```python
from build123d import *

# Parameters (mm, degrees)
CYLINDER016_R     = 1.75
CYLINDER016_DEPTH = 22
CYLINDER017_R     = 3
CYLINDER017_DEPTH = 22
CYLINDER015_R     = 1.75
CYLINDER015_DEPTH = 22
CYLINDER014_R     = 3
CYLINDER014_DEPTH = 22
CYLINDER013_R     = 1.75
CYLINDER013_DEPTH = 22
CYLINDER012_R     = 3
CYLINDER012_DEPTH = 22
CYLINDER011_R     = 1.75
CYLINDER011_DEPTH = 22
CYLINDER010_R     = 3
CYLINDER010_DEPTH = 22
CYLINDER009_R     = 0.5
CYLINDER009_DEPTH = 2
CYLINDER008_R     = 0.5
CYLINDER008_DEPTH = 2
BOX002_W          = 17.5
BOX002_H          = 10
BOX002_DEPTH      = 5
CYLINDER006_R     = 0.93
CYLINDER006_DEPTH = 10
CYLINDER007_R     = 2
CYLINDER007_DEPTH = 10
CYLINDER005_R     = 0.93
CYLINDER005_DEPTH = 10
CYLINDER004_R     = 2
CYLINDER004_DEPTH = 10
CYLINDER003_R     = 0.93
CYLINDER003_DEPTH = 10
CYLINDER002_R     = 2
CYLINDER002_DEPTH = 10
CYLINDER001_R     = 0.93
CYLINDER001_DEPTH = 10
CYLINDER_R        = 2
CYLINDER_DEPTH    = 10
BOX001_W          = 46
BOX001_H          = 46
BOX001_DEPTH      = 25
BOX_W             = 50
BOX_H             = 50
BOX_DEPTH         = 25
FILLET_R          = 1.5
FILLET001_R       = 1
FILLET002_R       = 0.5


with BuildPart() as cylinder008:
    # Cylinder016 → Cylinder016 (new body)
    with BuildSketch(Plane.XY):
        Circle(CYLINDER016_R)
    extrude(amount=CYLINDER016_DEPTH)


with BuildPart() as cut008:
    # Cylinder017 → Cylinder017 (new body)
    with BuildSketch(Plane.XY):
        Circle(CYLINDER017_R)
    extrude(amount=CYLINDER017_DEPTH)

    # Cut008: cut Cylinder008
    add(cylinder008.part, mode=Mode.SUBTRACT)


with BuildPart() as cut008_1:
    # Cut008 placement: moved
    add(cut008.part.moved(Location((41, 35, 0))))


with BuildPart() as cylinder007:
    # Cylinder015 → Cylinder015 (new body)
    with BuildSketch(Plane.XY):
        Circle(CYLINDER015_R)
    extrude(amount=CYLINDER015_DEPTH)


with BuildPart() as fusion007:
    # Cylinder014 → Cylinder014 (new body)
    with BuildSketch(Plane.XY):
        Circle(CYLINDER014_R)
    extrude(amount=CYLINDER014_DEPTH)

    # Cut009: cut Cylinder007
    add(cylinder007.part, mode=Mode.SUBTRACT)


with BuildPart() as fusion007_1:
    # Cut009 placement: moved
    add(fusion007.part.moved(Location((6, 35, 0))))

    # Fusion007: union Cut008
    add(cut008_1.part)


with BuildPart() as fusion007_2:
    # Fusion007 placement: moved
    add(fusion007_1.part.moved(Location((0, -35, 0))))


with BuildPart() as cylinder005:
    # Cylinder013 → Cylinder013 (new body)
    with BuildSketch(Plane.XY):
        Circle(CYLINDER013_R)
    extrude(amount=CYLINDER013_DEPTH)


with BuildPart() as cut007:
    # Cylinder012 → Cylinder012 (new body)
    with BuildSketch(Plane.XY):
        Circle(CYLINDER012_R)
    extrude(amount=CYLINDER012_DEPTH)

    # Cut007: cut Cylinder005
    add(cylinder005.part, mode=Mode.SUBTRACT)


with BuildPart() as cut007_1:
    # Cut007 placement: moved
    add(cut007.part.moved(Location((41, 35, 0))))


with BuildPart() as cylinder003:
    # Cylinder011 → Cylinder011 (new body)
    with BuildSketch(Plane.XY):
        Circle(CYLINDER011_R)
    extrude(amount=CYLINDER011_DEPTH)


with BuildPart() as pcb_platform:
    # Cylinder010 → Cylinder010 (new body)
    with BuildSketch(Plane.XY):
        Circle(CYLINDER010_R)
    extrude(amount=CYLINDER010_DEPTH)

    # Cut006: cut Cylinder003
    add(cylinder003.part, mode=Mode.SUBTRACT)


with BuildPart() as pcb_platform_1:
    # Cut006 placement: moved
    add(pcb_platform.part.moved(Location((6, 35, 0))))

    # Fusion005: union Cut007
    add(cut007_1.part)

    # Fusion008: union Fusion007
    add(fusion007_2.part)


with BuildPart() as pcb_platform_2:
    # Fusion008 placement: moved
    add(pcb_platform_1.part.moved(Location((1, 7, 0))))


with BuildPart() as cylinder001:
    # Cylinder009 → Cylinder009 (new body)
    with BuildSketch(Plane(origin=(13.5, 0, 0), x_dir=(1, 0, 0), z_dir=(0, 0, 1))):
        Circle(CYLINDER009_R)
    extrude(amount=CYLINDER009_DEPTH)


with BuildPart() as fusion004:
    # Cylinder008 → Cylinder008 (new body)
    with BuildSketch(Plane.XY):
        Circle(CYLINDER008_R)
    extrude(amount=CYLINDER008_DEPTH)

    # Fusion004: union Cylinder001
    add(cylinder001.part)


with BuildPart() as fusion004_1:
    # Fusion004 placement: moved
    add(fusion004.part.moved(Location((18, 5, 1))))


with BuildPart() as cube:
    # Box002 → Box002 (new body)
    with BuildSketch(Plane(origin=(16, 0, 2), x_dir=(1, 0, 0), z_dir=(0, 0, 1))):
        with Locations((8.75, 5)):
            Rectangle(BOX002_W, BOX002_H)
    extrude(amount=BOX002_DEPTH)


with BuildPart() as obj1:
    # Cylinder006 → Cylinder006 (new body)
    with BuildSketch(Plane(origin=(7, 10, 2), x_dir=(1, 0, 0), z_dir=(0, 0, 1))):
        Circle(CYLINDER006_R)
    extrude(amount=CYLINDER006_DEPTH)


with BuildPart() as obj2:
    # Cylinder007 → Cylinder007 (new body)
    with BuildSketch(Plane(origin=(7, 10, 0), x_dir=(1, 0, 0), z_dir=(0, 0, 1))):
        Circle(CYLINDER007_R)
    extrude(amount=CYLINDER007_DEPTH)

    # Cut004: cut obj1
    add(obj1.part, mode=Mode.SUBTRACT)


with BuildPart() as obj2_1:
    # Cut004 placement: moved
    add(obj2.part.moved(Location((37.64, 14.24, 0))))


with BuildPart() as obj3:
    # Cylinder005 → Cylinder005 (new body)
    with BuildSketch(Plane(origin=(7, 10, 2), x_dir=(1, 0, 0), z_dir=(0, 0, 1))):
        Circle(CYLINDER005_R)
    extrude(amount=CYLINDER005_DEPTH)


with BuildPart() as fusion001:
    # Cylinder004 → Cylinder004 (new body)
    with BuildSketch(Plane(origin=(7, 10, 0), x_dir=(1, 0, 0), z_dir=(0, 0, 1))):
        Circle(CYLINDER004_R)
    extrude(amount=CYLINDER004_DEPTH)

    # Cut003: cut obj3
    add(obj3.part, mode=Mode.SUBTRACT)


with BuildPart() as fusion001_1:
    # Cut003 placement: moved
    add(fusion001.part.moved(Location((37.64, -1, 0))))

    # Fusion001: union obj2
    add(obj2_1.part)


with BuildPart() as obj4:
    # Cylinder003 → Cylinder003 (new body)
    with BuildSketch(Plane(origin=(7, 10, 2), x_dir=(1, 0, 0), z_dir=(0, 0, 1))):
        Circle(CYLINDER003_R)
    extrude(amount=CYLINDER003_DEPTH)


with BuildPart() as obj5:
    # Cylinder002 → Cylinder002 (new body)
    with BuildSketch(Plane(origin=(7, 10, 0), x_dir=(1, 0, 0), z_dir=(0, 0, 1))):
        Circle(CYLINDER002_R)
    extrude(amount=CYLINDER002_DEPTH)

    # Cut002: cut obj4
    add(obj4.part, mode=Mode.SUBTRACT)


with BuildPart() as obj5_1:
    # Cut002 placement: moved
    add(obj5.part.moved(Location((-3, 14.24, 0))))


with BuildPart() as obj6:
    # Cylinder001 → Cylinder001 (new body)
    with BuildSketch(Plane(origin=(7, 10, 2), x_dir=(1, 0, 0), z_dir=(0, 0, 1))):
        Circle(CYLINDER001_R)
    extrude(amount=CYLINDER001_DEPTH)


with BuildPart() as nanoplatform:
    # Cylinder → Cylinder (new body)
    with BuildSketch(Plane(origin=(7, 10, 0), x_dir=(1, 0, 0), z_dir=(0, 0, 1))):
        Circle(CYLINDER_R)
    extrude(amount=CYLINDER_DEPTH)

    # Cut001: cut obj6
    add(obj6.part, mode=Mode.SUBTRACT)


with BuildPart() as nanoplatform_1:
    # Cut001 placement: moved
    add(nanoplatform.part.moved(Location((-3, -1, 0))))

    # Fusion: union obj5
    add(obj5_1.part)

    # Fusion002: union Fusion001
    add(fusion001_1.part)


with BuildPart() as nanoplatform_2:
    # Fusion002 placement: moved
    add(nanoplatform_1.part.moved(Location((0, 8, 0))))


with BuildPart() as obj7:
    # Box001 → Box001 (new body)
    with BuildSketch(Plane(origin=(2, 2, 2), x_dir=(1, 0, 0), z_dir=(0, 0, 1))):
        with Locations((23, 23)):
            Rectangle(BOX001_W, BOX001_H)
    extrude(amount=BOX001_DEPTH)


with BuildPart() as fillet002:
    # Box → Box (new body)
    with BuildSketch(Plane.XY):
        with Locations((25, 25)):
            Rectangle(BOX_W, BOX_H)
    extrude(amount=BOX_DEPTH)

    # Cut: cut obj7
    add(obj7.part, mode=Mode.SUBTRACT)

    # Fusion003: union NanoPlatform
    add(nanoplatform_2.part)

    # Cut005: cut Cube
    add(cube.part, mode=Mode.SUBTRACT)

    # Fusion006: union Fusion004
    add(fusion004_1.part)

    # Fusion009: union PCB_Platform
    add(pcb_platform_2.part)

    # Fillet
    fillet_edges = [fillet002.edges().sort_by_distance(p)[0] for p in [
        (0, 0, 12.5),
        (0, 50, 12.5),
        (50, 0, 12.5),
        (50, 50, 12.5),
    ]]
    fillet(fillet_edges, radius=FILLET_R)

    # Fillet001
    fillet001_edges = [fillet002.edges().sort_by_distance(p)[0] for p in [
        (0, 25, 0),
        (0.43934, 0.43934, 0),
        (0.43934, 49.56066, 0),
        (25, 0, 0),
        (25, 50, 0),
        (49.56066, 0.43934, 0),
        (49.56066, 49.56066, 0),
        (50, 25, 0),
    ]]
    fillet(fillet001_edges, radius=FILLET001_R)

    # Fillet002
    fillet002_edges = [fillet002.edges().sort_by_distance(p)[0] for p in [
        (24.75, 0, 7),
        (33.5, 0, 4.5),
        (24.75, 0, 2),
        (16, 0, 4.5),
    ]]
    fillet(fillet002_edges, radius=FILLET002_R)


solid = fillet002.part
```
Build history of the part. All positions in model axes, mm. A direction names the side the tool comes from. Give positions to 0.01 mm unless a question says otherwise; leave off trailing zeros. Loops run counter-clockwise (first coordinate to the right, second up) from the corner with the lowest first, then second, coordinate; pieces in that order, holes last.
Item 1: Slice it at A-A, the plane z = 19.75. Give the number of separate pieces and of enclosed holes in the cut face, and give its area (3 significant figures).
Answers follow:
separate pieces: 5
enclosed holes: 5
area: 457 mm2
Item 2: Pull direction Y, two halves, no side cores. Call faces 1 (the face through (0.43, 0.45, 13.17)), 2 (the face through (25, 50, 13)), 3 (the face through (7, 7, 2)): released by +Y, released by -Y, zero draft, split by the parting line, or undercut.
Answers follow:
face 1: released by -Y
face 2: released by +Y
face 3: undercut
Item 3: Slice it at D-D, the plane x = 42. List the corners of the cut face in (y, z).
Answers follow:
outline: (0, 1) arc R1 ccw to (1, 0) - (49, 0) arc R1 ccw to (50, 1) - (50, 25) - (48, 25) - (48, 2) - (45, 2) - (45, 22) - (43.75, 22) - (43.75, 2) - (40.25, 2) - (40.25, 22) - (39, 22) - (39, 2) - (10, 2) - (10, 22) - (8.75, 22) - (8.75, 2) - (5.25, 2) - (5.25, 22) - (4, 22) - (4, 2) - (2, 2) - (2, 25) - (0, 25) - close
Item 4: Drill centre lines: line 1 (Y direction, x = 7, z = 6.75); line 2 (Y direction, x = 46, z = 17.5). Where is each one in solid material? Low to high.
Answers follow:
line 1: y = 0 to 2, 4 to 5.25, 8.75 to 10, 39 to 40.25, 43.75 to 45, 48 to 50
line 2: y = 0 to 2, 48 to 50
Item 5: Slice it at B-B, the plane x = 25. List the corners of the cut face in (y, z).
Answers follow:
outline: (0, 1) arc R1 ccw to (1, 0) - (49, 0) arc R1 ccw to (50, 1) - (50, 25) - (48, 25) - (48, 2) - (0.5, 2) arc R0.5 ccw to (0, 1.5) - close; (0, 7.5) arc R0.5 ccw to (0.5, 7) - (2, 7) - (2, 25) - (0, 25) - close
Item 6: Flat gauge pins, fed straight in: pin 1 (1.2 mm diameter, centred on x = 3.5, y = 31.5, fed in from +Z); pin 2 (4.5 mm diameter, centred on x = 42, y = 7, fed in from +Z); pin 3 (10 mm diameter, centred on x = 32.5, y = 11, fed in from +Z). Where does each tip first touch, or does it go through?
Answers follow:
pin 1: stops at z = 10
pin 2: stops at z = 22
pin 3: stops at z = 2
Item 7: Which spindle directions (+Z, -Z, +X, -X, +Y, -Y) get a long thin tool onto all of the face, cutting with end or side? Do faces 4 (the face through (46, 32, 10)), 5 (the face through (23, 1, 25)). Say none if no direction does.
Answers follow:
face 4: +Z
face 5: +Z, +X, -X, +Y, -Y
Item 8: Slice it at C-C, the plane y = 11.5. List the corners of the cut face in (x, z).
Answers follow:
outline: (0, 1) arc R1 ccw to (1, 0) - (49, 0) arc R1 ccw to (50, 1) - (50, 25) - (48, 25) - (48, 2) - (2, 2) - (2, 25) - (0, 25) - close
